```python
from build123d import *

# Parameters (mm, degrees)
F0_W     = 50.8
F0_H     = 6.35
F1_DEPTH = 259.08
F2_W     = 50.8
F2_H     = 6.35
F3_ANGLE = -180
F4_W     = 50.8
F4_H     = 6.35
F5_ANGLE = 180
F7_DEPTH = 50.8


with BuildPart() as f1:
    # F0 (on Front) → F1 (new body)
    with BuildSketch(Plane.XZ):
        with Locations((-25.4, 3.175)):
            Rectangle(F0_W, F0_H)
    extrude(amount=F1_DEPTH)

    # F2 (on face) → F3 (revolve)
    with BuildSketch(Plane.XZ.offset(259.08)):
        with Locations((-25.4, 3.175)):
            Rectangle(F2_W, F2_H)
    revolve(axis=Axis((-25.4, -259.08, -25.4), (-1, 0, 0)), revolution_arc=F3_ANGLE)

    # F4 (on face) → F5 (revolve)
    with BuildSketch(Plane(origin=(0, 0, 0), x_dir=(-1, 0, 0), z_dir=(0, 1, 0))):
        with Locations((25.4, 3.175)):
            Rectangle(F4_W, F4_H)
    revolve(axis=Axis((-31.75, 0, -19.05), (-1, 0, 0)), revolution_arc=F5_ANGLE)

    # F6 (on face) → F7 (join)
    with BuildSketch(Plane(origin=(-50.8, 0, 0), x_dir=(0, -1, 0), z_dir=(-1, 0, 0))):
        Polygon((259.08, -50.8), (0, -38.1), (0, -44.45), (259.08, -57.15), align=None)
    extrude(amount=-F7_DEPTH)


solid = f1.part
```
Part model, mm, in its own coordinate system. A direction names the side the tool comes from. Round coordinates to 2 decimals unless told otherwise and drop trailing zeros. Write each loop counter-clockwise with the first axis right and the second up, starting at its lowest first coordinate (ties: lowest second). Pieces come first, ordered by that corner, then holes.
Item 1: Two-plate mould, pull along Z, no slides. Class faces 3 (the cylindrical face through (-25.044, -290.822, -24.702)), 4 (the flat face through (0, -132, -49)), 5 (the flat face through (-25.76, -131.35, -44.54)): +Z half, -Z half, draft (parallel to the pull), parting line (faces both ways), or undercut.
Results:
face 3: parting line
face 4: draft
face 5: undercut
Item 2: Cut at A-A, the plane x = -23. Give the cut face in (y, z).
Results:
outline: (-259.08, -57.15) - (0, -44.45) arc R25.4 ccw to (0, 6.35) - (-259.08, 6.35) arc R31.75 ccw to start; hole (-259.08, -50.8) - (0, -38.1) arc R19.05 ccw to (0, 0) - (-259.08, 0) arc R25.4 ccw to start
Item 3: Probe L1, parallel to Y at x = -36.5, z = -25; L2, parallel to Z at x = -6, y = -84.5; L3, parallel to Z at x = -19.5, y = -223.5. List the from-to ranges inside material, lowest first.
Results:
L1: y = -290.83 to -284.48, 18.1 to 24.69
L2: z = -48.59 to -42.24, 0 to 6.35
L3: z = -55.41 to -49.06, 0 to 6.35
Item 4: Cut at C-C, the plane y = -246. Give the cut face in (x, z), plus the area to 3 significant figures.
Results:
outline: (-50.8, -56.51) - (0, -56.51) - (0, -50.16) - (-50.8, -50.16) - close; (-50.8, 0) - (0, 0) - (0, 6.35) - (-50.8, 6.35) - close
area: 645 mm2
Item 5: Cut at B-B, the plane z = -11. Give the cut face in (x, y), plus the area to 3 significant figures.
Results:
outline: (-50.8, -287.38) - (0, -287.38) - (0, -280) - (-50.8, -280) - close; (-50.8, 17.27) - (0, 17.27) - (0, 24.09) - (-50.8, 24.09) - close
area: 721 mm2
Item 6: Which spindle directions (+Z, -Z, +X, -X, +Y, -Y) get a long thin tool onto all of the face, cutting with end or side? Do faces 1 (the flat face through (-25.76, -127.73, -50.71)), 2 (the flat face through (-26, -128, 0)). Say none if no direction does.
Results:
face 1: -Z, +X, -X, +Y
face 2: +X, -X
Item 7: Drop flat-ended pins along their axis: pin 1 Ø3 at (x, y) = (-37, -20) entering from -Z; pin 2 Ø6 at (x, z) = (-14, -16) entering from +Y; pin 3 Ø2 at (x, y) = (-38.5, -100) entering from -Z. Give the stop position or say it passes through.
Results:
pin 1: stops at z = -45.5
pin 2: stops at y = 25.4
pin 3: stops at z = -49.4
